from build123d import *

# Parameters (mm, degrees)
SKETCH1_R                                       = 12.446
SKETCH1_R_2                                     = 1.27
BOSS_EXTRUDE1_DEPTH                             = 17.272
CSK_FOR_M3_FLAT_HEAD_MACHINE_SCREW1_D           = 3.4
CSK_FOR_M3_FLAT_HEAD_MACHINE_SCREW1_CSINK_D     = 6.3
CSK_FOR_M3_FLAT_HEAD_MACHINE_SCREW1_CSINK_ANGLE = 90
SKETCH5_R                                       = 12.192
BOSS_EXTRUDE2_DEPTH                             = 30.734
SKETCH6_R                                       = 3.556
BOSS_EXTRUDE3_DEPTH                             = 2.54
SKETCH7_R                                       = 2.032
BOSS_EXTRUDE4_DEPTH                             = 9.906
SKETCH8_W                                       = 2.032
SKETCH8_H                                       = 0.254
CUT_EXTRUDE2_DEPTH                              = 9.906


with BuildPart() as part:
    # Sketch1 → Boss-Extrude1 (new body)
    with BuildSketch(Plane(origin=(0, 0, 0), x_dir=(1, 0, 0), z_dir=(0, 1, 0))):
        Circle(SKETCH1_R)
        with Locations((-9.017, 0)):
            Circle(SKETCH1_R_2, mode=Mode.SUBTRACT)
        with Locations((9.017, 0)):
            Circle(SKETCH1_R_2, mode=Mode.SUBTRACT)
    extrude(amount=BOSS_EXTRUDE1_DEPTH)

    # CSK for M3 Flat Head Machine Screw1 (through all)
    with Locations(Plane(origin=(0, 17.272, 0), x_dir=(1, 0, 0), z_dir=(0, 1, 0))):
        with Locations((0, 8.119865968), (0, -7.587036194)):
            CounterSinkHole(CSK_FOR_M3_FLAT_HEAD_MACHINE_SCREW1_D / 2, CSK_FOR_M3_FLAT_HEAD_MACHINE_SCREW1_CSINK_D / 2, counter_sink_angle=CSK_FOR_M3_FLAT_HEAD_MACHINE_SCREW1_CSINK_ANGLE)

    # Sketch5 → Boss-Extrude2 (add)
    with BuildSketch(Plane(origin=(0, 17.272, 0), x_dir=(1, 0, 0), z_dir=(0, 1, 0))):
        Circle(SKETCH5_R)
    extrude(amount=BOSS_EXTRUDE2_DEPTH)

    # Sketch6 → Boss-Extrude3 (add)
    with BuildSketch(Plane(origin=(0, 0, 0), x_dir=(1, 0, 0), z_dir=(0, 1, 0))):
        Circle(SKETCH6_R)
    extrude(amount=-BOSS_EXTRUDE3_DEPTH)

    # Sketch7 → Boss-Extrude4 (add)
    with BuildSketch(Plane(origin=(0, -2.54, 0), x_dir=(-1, 0, 0), z_dir=(0, -1, 0))):
        Circle(SKETCH7_R)
    extrude(amount=BOSS_EXTRUDE4_DEPTH)

    # Sketch8 → Cut-Extrude2 (cut)
    with BuildSketch(Plane(origin=(0, -12.446, 0), x_dir=(-1, 0, 0), z_dir=(0, -1, 0))):
        with Locations((0, -1.905)):
            Rectangle(SKETCH8_W, SKETCH8_H)
        with Locations((0, 1.905)):
            Rectangle(SKETCH8_W, SKETCH8_H)
    extrude(amount=-CUT_EXTRUDE2_DEPTH, mode=Mode.SUBTRACT)


solid = part.part
Source: CAD feature listing. Evaluate the final solid. Frame: model axes, mm. A direction names the side the tool comes from. Coordinates: 2 decimals unless noted, no trailing zeros. Loops run counter-clockwise (first coordinate to the right, second up) from the corner with the lowest first, then second, coordinate; pieces in that order, holes last. Notation, with made-up numbers: M 22,20 L 39,20 A30 ccw 39,48 Z; hole C -35.5,4.5 d10. An arc over 180 degrees is marked long. Answer in a Markdown table with one row per item.
Q1. Ray query, probe 1 along Z at (x, y) = (0, 5.25); probe 2 along X at (y, z) = (9.25, 0); probe 3 along Z at (x, y) = (1, 1). Return the intervals inside material, ascending. Write a range as from..to.
Answers below:
| item | result |
|---|---|
| probe 1 | z = -12.45..-9.82, -6.42..5.89, 9.29..12.45 |
| probe 2 | x = -12.45..-10.29, -7.75..7.75, 10.29..12.45 |
| probe 3 | z = -12.41..-9.49, -6.75..6.21, 8.96..12.41 |
Q2. Section A-A on x = 0. Return the cut outline in (y, z).
Answers below:
| item | result |
|---|---|
| outline | M -12.45,-1.78 L -2.54,-1.78 L -2.54,-3.56 L 0,-3.56 L 0,-6.42 L 15.82,-6.42 L 17.27,-4.97 L 17.27,-11.27 L 15.82,-9.82 L 0,-9.82 L 0,-12.45 L 17.27,-12.45 L 17.27,-12.19 L 48.01,-12.19 L 48.01,12.19 L 17.27,12.19 L 17.27,12.45 L 0,12.45 L 0,9.29 L 15.82,9.29 L 17.27,10.74 L 17.27,4.44 L 15.82,5.89 L 0,5.89 L 0,3.56 L -2.54,3.56 L -2.54,1.78 L -12.45,1.78 Z |
Q3. Draft query along X for faces 4 (the cylindrical face through (-2.03, -7.42, 0.03)), 5 (the flat face through (0, -12.446, 0)), 6 (the flat face through (-9, 17.272, 0)), 7 (the cylindrical face through (-0.77, -1.25, 3.47)). Return one class per face: pulls with the +X half, pulls with the -X half, needs draft (parallel to the pull), parting line crosses it, or undercut.
Answers below:
| item | result |
|---|---|
| face 4 | pulls with the -X half |
| face 5 | needs draft |
| face 6 | undercut |
| face 7 | parting line crosses it |
Q4. Section D-D on y = 32.5. Return the cut outline in (x, z), plus the area to 3 significant figures.
Answers below:
| item | result |
|---|---|
| outline | C 0,0 d24.38 |
| area | 467 mm^2 |
Q5. Section C-C on y = 3. Return the cut outline in (x, z), plus the area to 3 significant figures.
Answers below:
| item | result |
|---|---|
| outline | C 0,0 d24.89; hole C -9.02,0 d2.54; hole C 0,-8.12 d3.4; hole C 0,7.59 d3.4; hole C 9.02,0 d2.54 |
| area | 458 mm^2 |
Q6. First-contact query: pin 1 (1.9 mm diameter, centred on x = -1.5, z = 9, fed in from -Y); pin 2 (4 mm diameter, centred on y = -0.5, z = -8.5, fed in from -X); pin 3 (2 mm diameter, centred on x = 0, y = -5, fed in from -Z). Flat tips, straight axial feed; report the tip coordinate or a pass-through.
Answers below:
| item | result |
|---|---|
| pin 1 | stops at y = 0 |
| pin 2 | stops at x = -10.57 |
| pin 3 | stops at z = -1.78 |
Q7. Set-up query: faces 1 (the conical face through (-1, 16, 6)), 2 (the cylindrical face through (7.75, 8.52, -0.06)), 3 (the cylindrical face through (2.03, -7.42, -0.03)). Return all of +Z, -Z, +X, -X, +Y, -Y with unobstructed straight access to the full face (end or side cutting, diameter ignored); none if empty.
Answers below:
| item | result |
|---|---|
| face 1 | none |
| face 2 | -Y |
| face 3 | +X, -Y |
Q8. Section B-B on z = 0. Return the cut outline in (x, y), plus the area to 3 significant figures.
Answers below:
| item | result |
|---|---|
| outline | M -12.45,0 L -10.29,0 L -10.29,17.27 L -7.75,17.27 L -7.75,0 L -3.56,0 L -3.56,-2.54 L -2.03,-2.54 L -2.03,-12.45 L 2.03,-12.45 L 2.03,-2.54 L 3.56,-2.54 L 3.56,0 L 7.75,0 L 7.75,17.27 L 10.29,17.27 L 10.29,0 L 12.45,0 L 12.45,17.27 L 12.19,17.27 L 12.19,48.01 L -12.19,48.01 L -12.19,17.27 L -12.45,17.27 Z |
| area | 1,150 mm^2 |
